```python
from build123d import *

# Parameters (mm, degrees)
SKETCH_1_R          = 2
EXTRUDE_1_DEPTH     = 16
SKETCH_2_R          = 4
EXTRUDE_2_DEPTH     = 2.5
FILLET_1_R          = 1
CHAMFER_1_SIZE      = 0.5
SKETCH_3_W          = 4
SKETCH_3_H          = 1
SKETCH_3_W_2        = 1
SKETCH_3_H_2        = 4
CUT_EXTRUDE_1_DEPTH = 1
CHAMFER_2_SIZE      = 1


with BuildPart() as part:
    # 草图1 → 凸台-拉伸1 (new body)
    with BuildSketch(Plane(origin=(0, 0, 0), x_dir=(1, 0, 0), z_dir=(0, 1, 0))):
        with Locations(Location((0, 0, 0), (0, 0, 270))):
            Circle(SKETCH_1_R)
    extrude(amount=EXTRUDE_1_DEPTH)

    # 草图2 → 凸台-拉伸2 (add)
    with BuildSketch(Plane(origin=(0, 16, 0), x_dir=(1, 0, 0), z_dir=(0, 1, 0))):
        with Locations(Location((0, 0, 0), (0, 0, 270))):
            Circle(SKETCH_2_R)
    extrude(amount=EXTRUDE_2_DEPTH)

    # 圆角1
    fillet_1_edges = [part.edges().sort_by_distance(p)[0] for p in [
        (0, 18.5, -4),
    ]]
    fillet(fillet_1_edges, radius=FILLET_1_R)

    # 倒角1
    chamfer_1_edges = [part.edges().sort_by_distance(p)[0] for p in [
        (0, 0, -2),
    ]]
    chamfer(chamfer_1_edges, length=CHAMFER_1_SIZE)

    # 草图3 → 切除-拉伸-薄壁1 (cut)
    with BuildSketch(Plane(origin=(0, 18.5, 0), x_dir=(1, 0, 0), z_dir=(0, 1, 0))):
        Rectangle(SKETCH_3_W, SKETCH_3_H)
        Rectangle(SKETCH_3_W_2, SKETCH_3_H_2)
    extrude(amount=-CUT_EXTRUDE_1_DEPTH, mode=Mode.SUBTRACT)

    # 倒角2
    chamfer_2_edges = [part.edges().sort_by_distance(p)[0] for p in [
        (0, 17.5, 2),
        (2, 17.5, 0),
        (0, 17.5, -2),
        (-2, 17.5, 0),
    ]]
    chamfer(chamfer_2_edges, length=CHAMFER_2_SIZE - 0.0001)  # a hair under: the kernel refuses the full size


solid = part.part
```
Check sheet for the modelled part. Datum: model origin and axes. Units: mm. A direction names the side the tool comes from. Coordinates: 2 decimals unless noted, no trailing zeros. Write each loop counter-clockwise with the first axis right and the second up, starting at its lowest first coordinate (ties: lowest second). Pieces come first, ordered by that corner, then holes. Notation, with made-up numbers: M 75,-4 L 89,-4 A26 cw 89,29 Z; hole C 48.25,50 d9. An arc over 180 degrees is marked long. Use one line per item in the form item = value.
Item 1: Release check for a two-part mould opening along X. For faces 1 (the face through (-1, 18.5, 1)), 2 (the face through (0.5, 18, -1)), 3 (the face through (-2, 8, 0)) record: pulls with the +X half, pulls with the -X half, needs draft (parallel to the pull), parting line crosses it, or undercut.
Answer below:
face_1 = needs draft
face_2 = undercut
face_3 = parting line crosses it
Item 2: Gauge pin test, flat ends, axial feed: pin 1 Ø1.5 at (x, y) = (-2, 9) entering from +Z; pin 2 Ø0.5 at (y, z) = (18, -1) entering from +X; pin 3 Ø2 at (x, y) = (-1.5, 15.5) entering from -Z; pin 4 Ø1.6 at (x, z) = (0.5, 0) entering from +Y. Record the tip position at first contact, or that the pin passes through.
Answer below:
pin_1 = 1.56
pin_2 = 3.86
pin_3 = -3.95
pin_4 = 18.5
Item 3: Sectioned sample at C-C, the plane y = 2.75. Record the cut outline in (x, z).
Answer below:
outline = C 0,0 d4
Item 4: Material ranges on L1, parallel to Y at x = -2, z = -2.25; L2, parallel to X at y = 2.25, z = 0; L3, parallel to Y at x = 0.25, z = 0, recorded low to high. Write a range as from..to.
Answer below:
L1 = 16..18.5
L2 = -2..2
L3 = 0..17.5
Item 5: Set-up check for faces 4 (the face through (1, 18, 0.5)), 5 (the face through (-3.905, 16.74, -0.867)): record each of +Z, -Z, +X, -X, +Y, -Y from which the full face is reachable in a straight line by a thin tool's end or side.
Answer below:
face_4 = +Y
face_5 = +Y, -Y
